Autodesk Inventor part; units mm, degrees
ref_plane "YZ Plane" through (0, 0, 0) normal (1, 0, 0) x (0, 1, 0)
ref_plane "XZ Plane" through (0, 0, 0) normal (0, 1, 0) x (-1, 0, 0)
ref_plane "XY Plane" through (0, 0, 0) normal (0, 0, 1) x (1, 0, 0)
sketch "Sketch1" plane through (0, 0, 0) normal (0, 0, 1) x (1, 0, 0)
  line L0 (-40.5, 47.5) -> (40.5, 47.5)
  line L1 (42.5, 45.5) -> (42.5, -45.5)
  line L2 (40.5, -47.5) -> (-40.5, -47.5)
  line L3 (-42.5, -45.5) -> (-42.5, 45.5)
  arc A0 (-40.5, 47.5) -> (-42.5, 45.5) centre (-40.5, 45.5) ccw
  arc A1 (-42.5, -45.5) -> (-40.5, -47.5) centre (-40.5, -45.5) ccw
  arc A2 (40.5, -47.5) -> (42.5, -45.5) centre (40.5, -45.5) ccw
  arc A3 (42.5, 45.5) -> (40.5, 47.5) centre (40.5, 45.5) ccw
  line L4 (-50.5, 57.5) -> (50.5, 57.5)
  line L5 (52.5, 55.5) -> (52.5, -55.5)
  line L6 (50.5, -57.5) -> (-50.5, -57.5)
  line L7 (-52.5, -55.5) -> (-52.5, 55.5)
  arc A4 (-50.5, 57.5) -> (-52.5, 55.5) centre (-50.5, 55.5) ccw
  arc A5 (-52.5, -55.5) -> (-50.5, -57.5) centre (-50.5, -55.5) ccw
  arc A6 (50.5, -57.5) -> (52.5, -55.5) centre (50.5, -55.5) ccw
  arc A7 (52.5, 55.5) -> (50.5, 57.5) centre (50.5, 55.5) ccw
  point P0 (0, 0)
  point P1 (-42.5, 47.5)
  point P2 (42.5, -47.5)
  point P3 (42.5, 47.5)
  dimension "d0" = 85
  dimension "d1" = 95
  dimension "d2" = 47.5
  dimension "d3" = 42.5
  dimension "d4" = 2
  dimension "d5" = 10
  dimension "d6" = 10
  dimension "d7" = 10
  dimension "d8" = 10
  dimension "d9" = 2
extrude "chamberBase" add sketch "Sketch1" along normal blind 5 contours L0 A3 L1 A2 L2 A1 L3 A0 | L4 A7 L5 A6 L6 A5 L7 A4
sketch "Sketch2" plane through (0, 0, 5) normal (0, 0, 1) x (1, 0, 0)
  line L0 (-33, 40) -> (33, 40)
  line L1 (35, 38) -> (35, -38)
  line L2 (33, -40) -> (-33, -40)
  line L3 (-35, -38) -> (-35, 38)
  arc A0 (-33, 40) -> (-35, 38) centre (-33, 38) ccw
  arc A1 (-35, -38) -> (-33, -40) centre (-33, -38) ccw
  arc A2 (33, -40) -> (35, -38) centre (33, -38) ccw
  arc A3 (35, 38) -> (33, 40) centre (33, 38) ccw
  point P0 (0, 0)
  point P1 (-35, 40)
  point P2 (35, -40)
  point P3 (35, 40)
  dimension "d12" = 70
  dimension "d13" = 80
  dimension "d14" = 40
  dimension "d15" = 35
  dimension "d16" = 2
extrude "chamberWallExt" add sketch "Sketch2" along normal blind 50
sketch "Sketch3" plane through (0, 0, 55) normal (0, 0, 1) x (1, 0, 0)
  line L0 (-32, 37) -> (29, 37)
  line L1 (29, 37) -> (29, -37)
  line L2 (29, -37) -> (-32, -37)
  line L3 (-32, -37) -> (-32, 37)
  line L4 (-33, 40) -> (33, 40)
  line L5 (35, -38) -> (35, 38)
  line L6 (-33, -40) -> (33, -40)
  line L7 (-35, -38) -> (-35, 38)
  point P0 (0, 0)
  dimension "d19" = 3
  dimension "d21" = 3
  dimension "d46" = 3
  dimension "d47" = 6
extrude "chamberIntExt" cut sketch "Sketch3" against normal blind 37.5
sketch "Sketch4" plane through (29, -37, 55) normal (-1, 0, 0) x (0, 0, 1)
  line L0 (-5, 69.5) -> (-35, 69.5)
  line L1 (-35, 69.5) -> (-35, 4.5)
  line L2 (-35, 4.5) -> (-5, 4.5)
  line L3 (-5, 4.5) -> (-5, 69.5)
  line L4 (-50, -18.5) -> (-50, 92.5)
  point P0 (-55, 37)
  dimension "d25" = 65
  dimension "d26" = 30
  dimension "d27" = 32.5
  dimension "d28" = 45
extrude "rectCoverSlipMountExt" cut sketch "Sketch4" against normal blind 2
sketch "Sketch5" plane through (31, -37, 55) normal (-1, 0, 0) x (0, 0, 1)
  line L0 (-10, 64.5) -> (-30, 64.5)
  line L1 (-30, 64.5) -> (-30, 9.5)
  line L2 (-30, 9.5) -> (-10, 9.5)
  line L3 (-10, 9.5) -> (-10, 64.5)
  line L4 (-50, 92.5) -> (-50, -18.5)
  point P0 (-55, 37)
  dimension "d31" = 55
  dimension "d32" = 20
  dimension "d33" = 27.5
  dimension "d34" = 40
extrude "rectCoverSlipWindow" cut sketch "Sketch5" against normal up to surface (4 mm away)
sketch "Sketch7" plane through (35, -38, 5) normal (1, 0, 0) x (0, 0, -1)
  line L0 (-50, 3) -> (0, 3)
  line L1 (0, 3) -> (0, 73)
  line L2 (0, 73) -> (-50, 73)
  line L3 (-50, 73) -> (-50, 3)
  line L4 (-50, 0) -> (-50, 76)
  line L5 (0, 76) -> (0, 0)
  point P0 (5, 38)
  dimension "d42" = 70
  dimension "d43" = 35
extrude "illObjExt" cut sketch "Sketch7" against normal blind 2
sketch "Sketch8" plane through (-32, 37, 55) normal (0, -1, 0) x (1, 0, 0)
  line L0 (56.5, -32.5) -> (11.5, -32.5)
  line L1 (11.5, -32.5) -> (11.5, -7.5)
  line L2 (11.5, -7.5) -> (56.5, -7.5)
  line L3 (56.5, -7.5) -> (56.5, -32.5)
  line L4 (0, -37.5) -> (61, -37.5)
  line L5 (-18.5, -50) -> (82.5, -50)
  point P0 (32, -55)
  point P1 (61, -5)
  dimension "d48" = 25
  dimension "d49" = 45
  dimension "d52" = 42.5
  dimension "d109" = 4.5
extrude "viewingWindCoverSlipMount" cut sketch "Sketch8" against normal blind 2
sketch "Sketch9" plane through (-32, 39, 55) normal (0, -1, 0) x (1, 0, 0)
  line L0 (16.5, -11.5) -> (51.5, -11.5)
  line L1 (51.5, -11.5) -> (51.5, -28.5)
  line L2 (51.5, -28.5) -> (16.5, -28.5)
  line L3 (16.5, -28.5) -> (16.5, -11.5)
  line L4 (82.5, -50) -> (-18.5, -50)
  line L5 (56.5, -7.5) -> (56.5, -32.5)
  point P0 (32, -55)
  dimension "d55" = 35
  dimension "d56" = 17
  dimension "d58" = 38.5
  dimension "d110" = 5
extrude "viewingWindExt" cut sketch "Sketch9" against normal up to surface (1 mm away)
sketch "Sketch10" plane through (0, 0, 17.5) normal (0, 0, 1) x (1, 0, 0)
  circle A0 centre (0, -15) radius 2.825
  circle A1 centre (15, 0) radius 2.825
  circle A2 centre (0, 15) radius 2.825
  circle A3 centre (-15, 0) radius 2.825
  circle A4 centre (0, 0) radius 2.825
  dimension "d70" = 5.65
  dimension "d71" = 5.65
  dimension "d72" = 5.65
  dimension "d73" = 5.65
  dimension "d74" = 5.65
  dimension "d75" = 15
  dimension "d76" = 15
  dimension "d77" = 15
  dimension "d78" = 15
extrude "sampleHolderMagnets" cut sketch "Sketch10" against normal blind 2
sketch "Sketch13" plane through (0, 0, 0) normal (0, 0, -1) x (-1, 0, 0)
  circle A0 centre (0, 55) radius 1.325
  circle A1 centre (-50, 0) radius 1.325
  circle A2 centre (0, -55) radius 1.325
  circle A3 centre (0, 0) radius 1.325
  circle A4 centre (50, 0) radius 1.325
  dimension "d98" = 2.65
  dimension "d99" = 2.65
  dimension "d100" = 2.65
  dimension "d101" = 2.65
  dimension "d102" = 2.65
  dimension "d103" = 55
  dimension "d104" = 55
  dimension "d105" = 50
  dimension "d106" = 50
extrude "xyStageMount" cut sketch "Sketch13" against normal blind 2
equation "\"d6\" = d5"
equation "\"d7\" = d5"
equation "\"d8\" = d5"
equation "\"d21\" = d19"
equation "\"d46\" = d19"
equation "\"d71\" = d70"
equation "\"d72\" = d70"
equation "\"d73\" = d70"
equation "\"d74\" = d70"
equation "\"d76\" = d75"
equation "\"d77\" = d75"
equation "\"d78\" = d75"
equation "\"d99\" = d98"
equation "\"d100\" = d98"
equation "\"d101\" = d98"
equation "\"d102\" = d98"
properties part number "sampleChamber"
Geometry check sheet. Reference: the model listing, model coordinates, mm. A direction names the side the tool comes from. Give positions to 0.01 mm unless a question says otherwise; leave off trailing zeros. Loops run counter-clockwise (first coordinate to the right, second up) from the corner with the lowest first, then second, coordinate; pieces in that order, holes last. Notation, with made-up numbers: (28, 78.25) - (87, 78.25) arc R16 ccw to (87, 89.25) - close; hole circle Ø2 at (0, 42). An arc over 180 degrees is marked (long way). Use CSV: the item, a comma, the result in double quotes. Start each with the question number.
Q1. Go/stop test with flat-tipped pins: pin 1 Ø2 at (x, y) = (-38.5, 3.5) entering from +Z; pin 2 Ø4.5 at (x, y) = (15, 0) entering from +Z; pin 3 Ø4 at (y, z) = (-7, 30) entering from +X. Record where each tip stops, or that it passes through.
Q2. Section check D-D, the plane y = -25.5. Record the cut outline in (x, z), and give its area (3 significant figures).
Q3. Section check B-B, the plane x = 15. Record the cut outline in (y, z) (3 decimals).
Q4. Release check for a two-part mould opening along Y. For faces 6 (the face through (0, 40, 24)), 7 (the face through (35, 37, 30)), 8 (the face through (-1, -37, 37)) record: +Y half, -Y half, draft (parallel to the pull), parting line (faces both ways), or undercut.
Q5. Scan lines: probe 1 along Y at (x, z) = (0, 16.25) (3 decimals); probe 2 along Y at (x, z) = (0, 1.4) (3 decimals); probe 3 along Y at (x, z) = (32, 26.5). Record each from-to range of solid material in increasing order. Write a range as from..to.
Q6. Section check A-A, the plane y = 15. Record the cut outline in (x, z) (3 decimals), and give its area (3 significant figures).
Q7. Access from +Z, -Z, +X, -X, +Y, -Y to the whole of each face (thin tool, end or side, straight path). Record for faces 1 (the face through (-51.264, 0.398, 0.986)), 2 (the face through (-35, -1, 30)), 3 (the face through (-1, 57.5, 2)), 4 (the face through (-12, 1, 0)), 5 (the face through (29, 5.7, 50.2)).
Findings below:
1,pin 1,"stops at z = 5"
1,pin 2,"stops at z = 15.5"
1,pin 3,"stops at x = -32"
2,outline,"(-52.5, 0) - (52.5, 0) - (52.5, 5) - (33, 5) - (33, 25) - (31, 25) - (31, 20) - (29, 20) - (29, 17.5) - (-32, 17.5) - (-32, 55) - (-35, 55) - (-35, 5) - (-52.5, 5) - close; (29, 50) - (31, 50) - (31, 45) - (33, 45) - (33, 55) - (29, 55) - close"
2,area,"1,540 mm^2"
3,outline,"(-57.5, 0) - (57.5, 0) - (57.5, 5) - (40, 5) - (40, 26.5) - (39, 26.5) - (39, 22.5) - (37, 22.5) - (37, 17.5) - (2.825, 17.5) - (2.825, 15.5) - (-2.825, 15.5) - (-2.825, 17.5) - (-37, 17.5) - (-37, 55) - (-40, 55) - (-40, 5) - (-57.5, 5) - close; (37, 47.5) - (39, 47.5) - (39, 43.5) - (40, 43.5) - (40, 55) - (37, 55) - close"
4,face 6,"+Y half"
4,face 7,"draft"
4,face 8,"undercut"
5,probe 1,"y = -40..-17.825, -12.175..-2.825, 2.825..12.175, 17.825..40"
5,probe 2,"y = -57.5..-56.325, -53.675..-1.325, 1.325..53.675, 56.325..57.5"
5,probe 3,"y = -40..-27.5, 27.5..40"
6,outline,"(-52.5, 0) - (52.5, 0) - (52.5, 5) - (33, 5) - (33, 25) - (31, 25) - (31, 20) - (29, 20) - (29, 17.5) - (2.825, 17.5) - (2.825, 15.5) - (-2.825, 15.5) - (-2.825, 17.5) - (-32, 17.5) - (-32, 55) - (-35, 55) - (-35, 5) - (-52.5, 5) - close; (29, 50) - (31, 50) - (31, 45) - (33, 45) - (33, 55) - (29, 55) - close"
6,area,"1,530 mm^2"
7,face 1,"-Z"
7,face 2,"+Z, -X, +Y, -Y"
7,face 3,"+Z, -Z, +X, -X, +Y"
7,face 4,"-Z, +X, -X, +Y, -Y"
7,face 5,"+Z"
